Input: part model. Units: mm. Frame: model coordinates. A direction names the side the tool comes from. Coordinates: 2 decimals unless noted, no trailing zeros. Write each loop counter-clockwise with the first axis right and the second up, starting at its lowest first coordinate (ties: lowest second). Pieces come first, ordered by that corner, then holes. Notation, with made-up numbers: (89.25, -36) -> (115.25, -36) arc R14 cw to (115.25, -27) -> close; hole circle Ø10 at (17.25, 37). An arc over 180 degrees is marked (long way). One line per question, with ' | ' between items. Start each with the question number.
```python
from build123d import *

# Parameters (mm, degrees)
BASPROSKE_W         = 132.2299391
BASPROSKE_H         = 22
TOOTHCUT_DEPTH      = 136.840924593
TEETHCUTS_COUNT     = 20
TEETHCUTS_ANGLE     = 342
BORSKE_R            = 0.4
BORE_DEPTH          = 50.0000508
SKETCH1_R           = 22
SKETCH1_R_2         = 21.342673338
CUT_EXTRUDE1_DEPTH  = 136.778456297
SCALE1_SCALE        = 0.4
SKETCH6_R           = 5
BOSS_EXTRUDE3_DEPTH = 15.0233807
CUT_EXTRUDE2_DEPTH  = 10
CUT_EXTRUDE3_START  = -2
SKETCH8_R           = 5
SKETCH8_R_2         = 3
CUT_EXTRUDE3_DEPTH  = 2


with BuildPart() as part:
    # BasProSke → Base-Revolve (revolve)
    with BuildSketch(Plane(origin=(0, 0, 0), x_dir=(1, 0, 0), z_dir=(0, 1, 0)), mode=Mode.PRIVATE) as base_revolve_sk:
        with Locations((66.11496955, 11)):
            Rectangle(BASPROSKE_W, BASPROSKE_H)
    revolve(base_revolve_sk.sketch.rotate(Axis((-10, 0, 0), (1, 0, 0)), 180), axis=Axis((-10, 0, 0), (1, 0, 0)))

    # TooCutSke → ToothCut (cut, through all)
    with BuildSketch(Plane(origin=(0, 0, 0), x_dir=(0, 0, -1), z_dir=(1, 0, 0))):
        with BuildLine():
            ThreePointArc((0.986171591, 17.471189616), (0, 17.499), (-0.986171591, 17.471189616))
            ThreePointArc((-0.986171591, 17.471189616), (-1.626916196, 19.798789858), (-2.932850173, 21.829260982))
            ThreePointArc((-2.932850173, 21.829260982), (0, 22.0254), (2.932850173, 21.829260982))
            ThreePointArc((2.932850173, 21.829260982), (1.626916196, 19.798789858), (0.986171591, 17.471189616))
        make_face()
    toothcut = extrude(amount=TOOTHCUT_DEPTH, mode=Mode.SUBTRACT)

    # TeethCuts: ToothCut ×20 about axis
    teethcuts_axis = Axis((-10, 0, 0), (1, 0, 0))
    for i in range(1, TEETHCUTS_COUNT):
        add(toothcut.rotate(teethcuts_axis, i * TEETHCUTS_ANGLE / (TEETHCUTS_COUNT - 1)), mode=Mode.SUBTRACT)

    # BorSke → Bore (cut, symmetric)
    with BuildSketch(Plane(origin=(0, 0, 0), x_dir=(0, 0, -1), z_dir=(1, 0, 0))):
        Circle(BORSKE_R)
    extrude(amount=BORE_DEPTH, both=True, mode=Mode.SUBTRACT)

    # Sketch1 → Cut-Extrude1 (cut, through all)
    with BuildSketch(Plane(origin=(132.2299391, 0, 0), x_dir=(0, 0, -1), z_dir=(1, 0, 0))):
        Circle(SKETCH1_R)
        Circle(SKETCH1_R_2, mode=Mode.SUBTRACT)
    extrude(amount=-CUT_EXTRUDE1_DEPTH, mode=Mode.SUBTRACT)


with BuildPart() as part_1:
    # Scale1: scaled about (0, 0, 0)
    add(part.part.scale(SCALE1_SCALE))

    # Sketch6 → Boss-Extrude3 (add)
    with BuildSketch(Plane(origin=(52.89197564, 0, 0), x_dir=(0, 0, -1), z_dir=(1, 0, 0))):
        with Locations(Location((0, 0, 0), (0, 0, 180))):
            Circle(SKETCH6_R)
    extrude(amount=BOSS_EXTRUDE3_DEPTH)

    # Sketch7 → Cut-Extrude2 (cut)
    with BuildSketch(Plane.ZY):
        with BuildLine():
            Line((2.5, 0), (2.5, 4.330127019))
            ThreePointArc((2.5, 4.330127019), (-5, 0), (2.5, -4.330127019))
            Line((2.5, -4.330127019), (2.5, 0))
        make_face()
    extrude(amount=-CUT_EXTRUDE2_DEPTH, mode=Mode.SUBTRACT)

    # Sketch8 → Cut-Extrude3 (cut)
    with BuildSketch(Plane(origin=(65.91535634, 0, 0), x_dir=(0, 0, -1), z_dir=(1, 0, 0)).offset(CUT_EXTRUDE3_START)):
        with Locations(Location((0, 0, 0), (0, 0, 180))):
            Circle(SKETCH8_R)
        Circle(SKETCH8_R_2, mode=Mode.SUBTRACT)
    extrude(amount=CUT_EXTRUDE3_DEPTH, mode=Mode.SUBTRACT)


solid = part_1.part
```
1) Section A-A, the plane x = 62.5. Return loops of the section in (y, z).
2) First-contact query: P1, Ø8, axis at x = 34.5, z = 4, coming from the +Y side; P2, Ø10, axis at x = 58, z = 3, coming from the +Y side; P3, Ø4, axis at x = 50.5, z = -5, coming from the +Y side. Flat tips, straight axial feed; report the tip coordinate or a pass-through.
3) Access query for faces 1 (the face through (58, 0, -5)), 2 (the face through (26.08, -7.58, -1.84)), 3 (the face through (26.076, -2.955, 7.201)). Directions: +Z, -Z, +X, -X, +Y, -Y. A direction counts if a zero-diameter tool reaches every point of the face in a straight line with its end or side. Return the directions, or none.
4) Pull-direction query (Z, two-part tool) for faces 4 (the face through (0, 0, 4)), 5 (the face through (26.076, 6.645, 4.094)), 6 (the face through (26.08, 2.97, 7.22)), 7 (the face through (26.08, 7.58, 1.84)); classes: released by +Z, released by -Z, zero draft, split by the parting line, or undercut.
5) Ray query, line 1 (X direction, y = 1.25, z = 4.25); line 2 (X direction, y = 4.5, z = -0.25); line 3 (X direction, y = 3, z = 4.75). Return the intervals inside material, ascending.
Answer block:
1) outline: circle Ø10 at (0, 0)
2) P1: stops at y = 8.48 | P2: stops at y = 5 | P3: stops at y = 7.77
3) face 1: +X | face 2: +X, -X | face 3: +Z, +X, -X
4) face 4: zero draft | face 5: undercut | face 6: released by +Z | face 7: undercut
5) line 1: x = 0 to 63.92, 65.92 to 67.92 | line 2: x = 10 to 63.92, 65.92 to 67.92 | line 3: x = 0 to 52.89
